Could you check a few things on this model? Use its own coordinates, in mm. A direction names the side the tool comes from. Give positions to 0.01 mm unless a question says otherwise; leave off trailing zeros. Write each loop counter-clockwise with the first axis right and the second up, starting at its lowest first coordinate (ties: lowest second). Pieces come first, ordered by that corner, then holes. Notation, with made-up numbers: M 31.25,-34.5 L 81.25,-34.5 A13 ccw 81.25,-12.5 Z; hole C 22,66.25 d2. An arc over 180 degrees is marked long. Write each question's results on one line, items separated by ' | '. Start each with the question number.
Autodesk Inventor part; units mm, degrees
ref_plane "YZ Plane" through (0, 0, 0) normal (1, 0, 0) x (0, 1, 0)
ref_plane "XZ Plane" through (0, 0, 0) normal (0, 1, 0) x (-1, 0, 0)
ref_plane "XY Plane" through (0, 0, 0) normal (0, 0, 1) x (1, 0, 0)
sketch "Sketch1" plane through (0, 0, 0) normal (0, 1, 0) x (-1, 0, 0)
  line L0 (0, 0) -> (84, 0)
  line L1 (84, 0) -> (84, -156)
  line L2 (0, -156) -> (0, 0)
  line L3 (0, 0) -> (3, 0) construction
  line L4 (3, 0) -> (3, -3) construction
  line L5 (3, -3) -> (0, -3) construction
  line L6 (0, -3) -> (0, 0) construction
  line L7 (84, -153) -> (84, -156) construction
  line L8 (3, -3) -> (30, -3)
  line L9 (30, -3) -> (30, -73)
  line L10 (30, -73) -> (3, -73)
  line L11 (3, -73) -> (3, -3)
  line L12 (78, -153) -> (54, -153)
  line L13 (54, -153) -> (54, -83)
  line L14 (54, -83) -> (81, -83)
  line L15 (81, -83) -> (81, -153)
  line L16 (0, -153) -> (0, -156) construction
  line L17 (84, 0) -> (81, 0) construction
  line L18 (81, 0) -> (81, -3) construction
  line L19 (81, -3) -> (84, -3) construction
  line L20 (84, -3) -> (84, 0) construction
  line L21 (81, -3) -> (54, -3)
  line L22 (54, -3) -> (54, -73)
  line L23 (54, -73) -> (81, -73)
  line L24 (81, -73) -> (81, -3)
  line L25 (6, -153) -> (30, -153)
  line L26 (30, -153) -> (30, -83)
  line L27 (30, -83) -> (3, -83)
  line L28 (3, -83) -> (3, -153)
  line L29 (30, -3) -> (33, -3) construction
  line L30 (54, -153) -> (51, -153) construction
  line L31 (33, -3) -> (51, -3)
  line L32 (51, -153) -> (33, -153)
  line L33 (3, -73) -> (3, -76) construction
  line L34 (81, -83) -> (81, -80) construction
  line L35 (81, -76) -> (81, -80)
  line L36 (3, -80) -> (3, -76)
  line L37 (33, -153) -> (33, -80)
  line L38 (33, -76) -> (33, -3)
  line L39 (3, -76) -> (33, -76)
  line L40 (51, -76) -> (81, -76)
  line L41 (81, -80) -> (51, -80)
  line L42 (33, -80) -> (3, -80)
  line L43 (51, -3) -> (51, -76)
  line L44 (51, -80) -> (51, -153)
  line L45 (6, -153) -> (78, -153)
  line L46 (3, -153) -> (6, -153)
  line L47 (6, -156) -> (3, -156)
  line L48 (81, -153) -> (78, -153)
  line L49 (78, -156) -> (81, -156)
  line L50 (6, -156) -> (78, -156)
  line L51 (81, -156) -> (84, -156)
  line L52 (3, -156) -> (0, -156)
  dimension "d1" = 156
  dimension "d12" = 3
  dimension "d13" = 3
  dimension "d15" = 70
  dimension "d17" = 70
  dimension "d66" = 3
  dimension "d68" = 3
extrude "Extrusion1" add sketch "Sketch1" along normal blind 23
sketch "Sketch5" plane through (0, 0, 0) normal (1, 0, 0) x (0, 0, -1)
  circle A0 centre (16.6, 11.5) radius 3.5
  circle A1 centre (139.4, 11.5) radius 3.5
  line L0 (153, 23) -> (83, 23)
  line L1 (156, 0) -> (0, 0)
  line L2 (16.6, 11.5) -> (51.6, 11.5)
  line L3 (139.4, 11.5) -> (104.4, 11.5)
  line L4 (51.6, 23) -> (104.4, 23)
  line L5 (104.4, 23) -> (104.4, 0)
  line L6 (104.4, 0) -> (51.6, 0)
  line L7 (51.6, 0) -> (51.6, 23)
  point P0 (162, 0)
  dimension "d97" = 35
  dimension "d98" = 35
extrude "Extrusion6" add sketch "Sketch5" along normal blind 21 contours L7 L4 L0 L5 L1
sketch "Sketch6" plane through (0, 23, 0) normal (0, 1, 0) x (1, 0, 0)
  line L0 (0, 51.6) -> (21, 51.6)
  line L1 (21, 51.6) -> (18, 51.6)
  line L2 (18, 51.6) -> (18, 54.6)
  line L3 (18, 54.6) -> (21, 54.6)
  line L4 (21, 54.6) -> (21, 51.6)
  line L5 (0, 104.4) -> (21, 104.4)
  line L6 (21, 104.4) -> (18, 104.4)
  line L7 (18, 104.4) -> (18, 101.4)
  line L8 (18, 101.4) -> (21, 101.4)
  line L9 (21, 101.4) -> (21, 104.4)
  line L10 (18, 54.6) -> (0, 54.6)
  line L11 (18, 54.6) -> (18, 101.4)
  line L12 (18, 101.4) -> (0, 101.4)
  line L13 (0, 54.6) -> (0, 101.4)
  line L14 (-84, 156) -> (-84, 0)
  line L15 (-84, 54.6) -> (-102, 54.6)
  line L16 (-84, 54.6) -> (-66, 54.6) construction
  line L17 (-102, 54.6) -> (-102, 101.4)
  line L18 (-102, 101.4) -> (-84, 101.4)
  line L19 (-84, 101.4) -> (-84, 104.4)
  line L20 (-84, 104.4) -> (-105, 104.4)
  line L21 (-105, 104.4) -> (-105, 51.6)
  line L22 (-105, 51.6) -> (-84, 51.6)
  line L23 (-84, 51.6) -> (-84, 54.6)
  point P0 (0, 0)
  point P1 (21, 49.6)
  point P2 (21, 106.4)
  dimension "d99" = 3
  dimension "d100" = 3
  dimension "d101" = 3
  dimension "d102" = 3
  dimension "d112" = 18
  dimension "d113" = 180
  dimension "d114" = 3
  dimension "d115" = 21
extrude "Extrusion7" cut sketch "Sketch6" against normal up to surface (23 mm away) contours L10 L13 L12 L11
extrude "Extrusion10" add sketch "Sketch6" against normal up to surface (23 mm away) contours L14 L18 L17 L15 L22 L21 L20
sketch "Sketch7" plane through (21, 0, 0) normal (1, 0, 0) x (0, 0, -1)
  line L0 (51.6, 0) -> (104.4, 0)
  circle A0 centre (91, 11.5) radius 8
  circle A1 centre (65, 11.5) radius 8
  line L1 (104.4, 23) -> (104.4, 0)
  line L2 (104.4, 23) -> (91, 23)
  line L3 (91, 23) -> (91, 11.5)
  line L4 (91, 11.5) -> (104.4, 11.5)
  line L5 (104.4, 11.5) -> (104.4, 23)
  circle A2 centre (91, 11.5) radius 8
  circle A3 centre (65, 11.5) radius 8
  point P0 (0, 0)
  dimension "d108" = 16
  dimension "d109" = 16
  dimension "d118" = 13.4
  dimension "d119" = 11.5
extrude "Extrusion9" cut sketch "Sketch7" against normal up to surface (3 mm away) contours L4 L3 A0 | A0 L3 L4 | A1
sketch "Sketch9" plane through (-105, 23, -104.4) normal (-1, 0, 0) x (0, 0, 1)
  line L0 (0, 0) -> (0, -23)
  line L1 (0, 0) -> (13.4, 0)
  line L2 (13.4, 0) -> (13.4, -11.5)
  line L3 (13.4, -11.5) -> (0, -11.5)
  line L4 (0, -11.5) -> (0, 0)
  circle A0 centre (13.4, -11.5) radius 8
  line L5 (0, 0) -> (52.8, 0)
  line L6 (52.8, 0) -> (39.4, 0)
  line L7 (39.4, 0) -> (39.4, -11.5)
  line L8 (39.4, -11.5) -> (52.8, -11.5)
  line L9 (52.8, -11.5) -> (52.8, 0)
  circle A1 centre (39.4, -11.5) radius 8
  point P0 (104.4, -23)
  dimension "d120" = 13.4
  dimension "d121" = 11.5
  dimension "d122" = 16
  dimension "d123" = 13.4
  dimension "d124" = 11.5
  dimension "d125" = 16
extrude "Extrusion11" cut sketch "Sketch9" against normal blind 10 contours A0 L2 L3 | L3 L2 A0 | A1 L8 L7 | L7 L8 A1
sketch "Sketch10" plane through (-84, 0, 0) normal (0, 0, 1) x (1, 0, 0)
  line L0 (25, 23) -> (25, 0)
  line L1 (0, 0) -> (84, 0)
  line L2 (25, 0) -> (22, 0)
  line L3 (22, 0) -> (22, 23)
  line L4 (22, 23) -> (25, 23)
  line L5 (59, 23) -> (59, 0)
  line L6 (81, 0) -> (54, 0)
  line L7 (59, 0) -> (62, 0)
  line L8 (62, 0) -> (62, 23)
  line L9 (62, 23) -> (59, 23)
  point P0 (0, 23)
  point P1 (84, 23)
  dimension "d128" = 25
  dimension "d129" = 3
  dimension "d130" = 25
  dimension "d131" = 3
extrude "Extrusion12" add sketch "Sketch10" along normal blind 23
sketch "Sketch11" plane through (-62, 0, 0) normal (-1, 0, 0) x (0, 0, 1)
  line L0 (0, 0) -> (23, 0)
  line L1 (23, 23) -> (20, 23)
  line L2 (20, 23) -> (20, 0)
  line L3 (20, 0) -> (23, 0)
  line L4 (23, 0) -> (23, 23)
  dimension "d134" = 3
extrude "Extrusion13" add sketch "Sketch11" along normal blind 47.5 and the other way blind 87.5
sketch "Sketch12" plane through (-84, 0, 23) normal (0, 0, 1) x (1, 0, 0)
  line L0 (109.5, 23) -> (62, 23)
  line L1 (109.5, 23) -> (71.4, 23)
  line L2 (71.4, 23) -> (71.4, 0)
  line L3 (-25.5, 0) -> (109.5, 0)
  line L4 (109.5, 0) -> (62, 0)
  line L5 (71.4, 23) -> (68.4, 23)
  line L6 (68.4, 23) -> (68.4, 0)
  line L7 (68.4, 0) -> (71.4, 0)
  line L8 (71.4, 0) -> (71.4, 23)
  line L9 (12.6, 23) -> (12.6, 0)
  line L10 (22, 0) -> (-25.5, 0)
  line L11 (12.6, 23) -> (15.6, 23)
  line L12 (15.6, 23) -> (15.6, 0)
  line L13 (15.6, 0) -> (12.6, 0)
  line L14 (12.6, 0) -> (12.6, 23)
  point P0 (84, 0)
  point P1 (-25.5, 23)
  point P2 (15.6, 0)
  dimension "d139" = 38.1
  dimension "d140" = 3
  dimension "d141" = 38.1
  dimension "d142" = 3
extrude "Extrusion14" add sketch "Sketch12" along normal blind 21
sketch "Sketch13" plane through (-71.4, 0, 23) normal (-1, 0, 0) x (0, 0, 1)
  line L0 (0, 23) -> (21, 23)
  line L1 (0, 0) -> (21, 0)
  line L2 (21, 23) -> (18, 23)
  line L3 (18, 23) -> (18, 0)
  line L4 (18, 0) -> (21, 0)
  line L5 (21, 0) -> (21, 23)
  point P0 (-23, 0)
  point P1 (18, 23)
  dimension "d145" = 3
extrude "Extrusion15" add sketch "Sketch13" against normal up to surface (58.8 mm away)
sketch "Sketch14" plane through (-84, 0, 44) normal (0, 0, 1) x (1, 0, 0)
  line L0 (71.4, 23) -> (54.6, 23)
  line L1 (54.6, 23) -> (54.6, 11.5)
  line L2 (54.6, 11.5) -> (71.4, 11.5)
  line L3 (71.4, 11.5) -> (71.4, 23)
  circle A0 centre (54.6, 11.5) radius 8
  line L4 (71.4, 23) -> (12.6, 23)
  line L5 (12.6, 23) -> (29.4, 23)
  line L6 (29.4, 23) -> (29.4, 11.5)
  line L7 (29.4, 11.5) -> (12.6, 11.5)
  line L8 (12.6, 11.5) -> (12.6, 23)
  circle A1 centre (29.4, 11.5) radius 8
  point P0 (84, 0)
  dimension "d148" = 16.8
  dimension "d149" = 11.5
  dimension "d150" = 16
  dimension "d151" = 16.8
  dimension "d152" = 11.5
  dimension "d153" = 16
extrude "Extrusion16" cut sketch "Sketch14" against normal blind 10 contours A0 L2 L1 | L1 L2 A0 | A1 L7 L6 | L6 L7 A1
properties part number "Motorcompartiment"
Q1. Please list where these lines run through material, in increasing order: line 1 (X direction, y = 21, z = -145); line 2 (Z direction, x = -103.9, y = 11.5); line 3 (Z direction, x = -85.5, y = 1.75). Write a range as [from, to].
Q2. If we mould it in two halves opening along X, with no side actions, what happens to faces 6 (the face through (-105, 12, -78)), 7 (the face through (-15.6, 12, 32)), 8 (the face through (-17, 11, -73)), 9 (the face through (6, 12, 23))? For each: pulls with the +X half, pulls with the -X half, needs draft (parallel to the pull), parting line crosses it, or undercut.
Q3. If we section it at A-A (x = -88.5): Please give me the cut outline in (y, z).
Q4. I'm going to push flat-ended pins straight in: P1, Ø2, axis at y = 11.5, z = 2.5, coming from the +X side; P2, Ø7, axis at y = 15, z = -116.5, coming from the -X side; P3, Ø10.5, axis at x = -94, y = 17, coming from the +Z side. Where does each tip first touch, or does it pass through?
Q5. If we section it at D-D (z = -132): Please give me the cut outline in (x, y), plus the area to 3 significant figures.
Q6. For faces 1 (the face through (19.521, 6.632, -58.651)), 2 (the face through (21, 12, -78)), 3 (the face through (-95, 12, -51.6)), 4 (the face through (-30, 11, -118)), 5 (the face through (-22, 11, 10)), which set-ups out of +Z, -Z, +X, -X, +Y, -Y let a thin tool reach every point of the face, with its end or its side?
Q7. If we section it at B-B (z = -91): Count the separate pieces of the cut face and the enclosed holes in it, plus the area to 3 significant figures.
Q8. If we section it at C-C (z = 14.5): Please give me the cut outline in (x, y).
Determined:
1) line 1: x = [-84, -81], [-54, -51], [-33, -30], [-3, 0] | line 2: z = [-104.4, -99], [-83, -73], [-57, -51.6], [20, 23] | line 3: z = [-104.4, -101.4], [-54.6, -51.6], [20, 23]
2) face 6: pulls with the -X half | face 7: undercut | face 8: undercut | face 9: needs draft
3) outline: M 0,-104.4 L 23,-104.4 L 23,-101.4 L 0,-101.4 Z; M 0,-54.6 L 23,-54.6 L 23,-51.6 L 0,-51.6 Z; M 0,20 L 23,20 L 23,23 L 0,23 Z
4) P1: stops at x = -22 | P2: stops at x = -84 | P3: stops at z = 23
5) outline: M -84,0 L -81,0 L -81,23 L -84,23 Z; M -54,0 L -51,0 L -51,23 L -54,23 Z; M -33,0 L -30,0 L -30,23 L -33,23 Z; M -3,0 L 0,0 L 0,23 L -3,23 Z | area: 276 mm²
6) face 1: +X | face 2: -Z, +X, +Y, -Y | face 3: -X, +Y, -Y | face 4: +Y, -Y | face 5: +X, +Y, -Y
7) separate pieces: 8 | enclosed holes: 0 | area: 318 mm²
8) outline: M -62,0 L -59,0 L -59,23 L -62,23 Z; M -25,0 L -22,0 L -22,23 L -25,23 Z
